Autodesk Inventor part; units mm, degrees
ref_plane "YZ Plane" through (0, 0, 0) normal (1, 0, 0) x (0, 1, 0)
ref_plane "XZ Plane" through (0, 0, 0) normal (0, 1, 0) x (-1, 0, 0)
ref_plane "XY Plane" through (0, 0, 0) normal (0, 0, 1) x (1, 0, 0)
sketch "Sketch1" plane through (0, 0, 0) normal (0, 1, 0) x (-1, 0, 0)
  line L0 (0, 0) -> (-3.05, 0)
  line L1 (-3.05, 0) -> (-3.05, -7.62)
  line L2 (-3.05, -7.62) -> (0, -7.62)
  line L3 (0, -7.62) -> (0, 0)
  line L4 (0, 0) -> (-0.635, 0)
  line L5 (-0.635, 0) -> (-0.635, 13.97)
  line L6 (-0.635, 13.97) -> (0, 13.97)
  line L7 (0, 13.97) -> (0, 0)
  line L8 (-0.635, 13.97) -> (0, 17.5713)
  line L9 (-0.635, 13.97) -> (3.0218, 13.97) construction
  line L10 (0, 17.5713) -> (0, 13.97)
  dimension "d0" = 3.05
  dimension "d1" = 7.62
  dimension "d2" = 0.635
  dimension "d3" = 13.97
  dimension "d13" = 80
  dimension "d14" = 10
  dimension "d15" = 17.5713
  dimension "d16" = 25.1913
revolve "Revolution1" add sketch "Sketch1" angle 360 about axis through (0, 0, 13.97) along (0, 0, -1)
sketch "Sketch2" plane through (0, 0, -7.62) normal (0, 0, -1) x (-1, 0, 0)
  circle A0 centre (0, 0) radius 3.05
  circle A1 centre (0, 0) radius 1.5
  dimension "d5" = 3
extrude "Extrusion1" cut sketch "Sketch2" against normal blind 3.25 contours A1
chamfer "Chamfer1" distance 1.143 angle 45 1 edges at (-3.05, 0, 0)
chamfer "Chamfer2" distance 0.254 angle 45 1 edges at (-3.05, 0, -7.62)
thread "Thread2"
properties part number "carbide_probe_30deg_tip_r02" material "Steel, High Strength, Low Alloy"
Input: part model. Units: mm. Frame: model coordinates. A direction names the side the tool comes from. Round coordinates to 2 decimals unless told otherwise and drop trailing zeros. Loops run counter-clockwise (first coordinate to the right, second up) from the corner with the lowest first, then second, coordinate; pieces in that order, holes last. Notation, with made-up numbers: (-10, 20) -> (30, 20) arc R31 ccw to (30, 56) -> close; hole circle Ø4 at (-18.5, 25). An arc over 180 degrees is marked (long way). One line per item, written item: value.
(1) Section A-A (z = -5.5). Return the cut outline in (x, y), plus the area to 3 significant figures.
Geometry check:
outline: circle Ø6.1 at (0, 0); hole circle Ø3 at (0, 0)
area: 22.2 mm2
(2) Pin query (flat end, axial travel): pin 1 (2 mm diameter, centred on x = -1, z = 1.5, fed in from -Y) (3 decimals); pin 2 (1 mm diameter, centred on y = -1.5, z = 12, fed in from -X). Return the tip coordinate at first contact, or that it passes through.
Geometry check:
pin 1: y = -0.635
pin 2: through
(3) Material intervals for line 1 (Y direction, x = 0, z = -5.8); line 2 (Z direction, x = -0.5, y = 1); line 3 (Y direction, x = -1.25, z = -5.5), sorted ascending. Write a range as [from, to].
Geometry check:
line 1: [-3.05, -1.5], [1.5, 3.05]
line 2: [-4.37, 0]
line 3: [-2.78, -0.83], [0.83, 2.78]
(4) Section B-B (z = 2). Return the cut outline in (x, y) (3 decimals).
Geometry check:
outline: circle Ø1.27 at (0, 0)
(5) Set-up query: faces 4 (the face through (1.5, 0.07, -6.02)), 5 (the face through (-3.047, -0.134, -4.298)). Return all of +Z, -Z, +X, -X, +Y, -Y with unobstructed straight access to the full face (end or side cutting, diameter ignored); none if empty.
Geometry check:
face 4: -Z
face 5: +Z, -Z
(6) Mould query, pull axis X, two halves, no side actions, for faces 1 (the face through (0, 1, 0)), 2 (the face through (-0.08, 0.63, 7.08)), 3 (the face through (0, 0, -4.37)). Classes: pulls with the +X half, pulls with the -X half, needs draft (parallel to the pull), parting line crosses it, or undercut.
Geometry check:
face 1: needs draft
face 2: parting line crosses it
face 3: undercut
